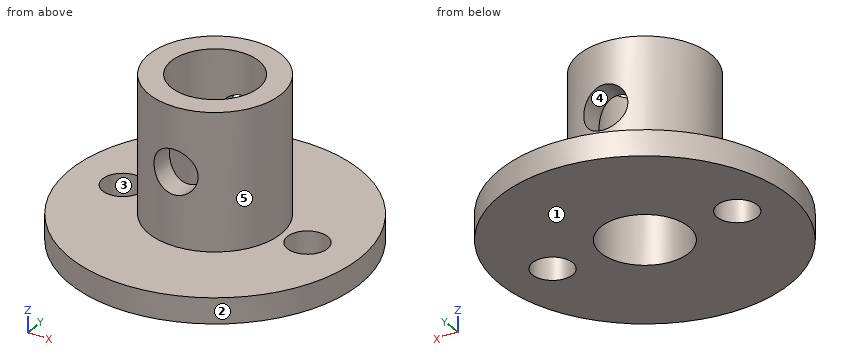
```python
from build123d import *

# Parameters (mm, degrees)
SKETCH1_W               = 10.16
SKETCH1_H               = 1.651
CUT_EXTRUDE1_DEPTH      = 20.458372876
CUT_EXTRUDE1_DEPTH_BACK = 20.458372876
SKETCH2_R               = 1.651
CUT_EXTRUDE2_DEPTH      = 19.338201985
CUT_EXTRUDE2_DEPTH_BACK = 19.338201985
SKETCH3_R               = 1.5


with BuildPart() as part:
    # Sketch1 → Revolve1 (revolve)
    with BuildSketch(Plane(origin=(0, 0, 0), x_dir=(0, 0, -1), z_dir=(1, 0, 0)), mode=Mode.PRIVATE) as revolve1_sk:
        with Locations((-6.985, 4.0894)):
            Rectangle(SKETCH1_W, SKETCH1_H)
        Polygon((-1.905, 10.795), (-1.905, 4.9149), (-1.905, 3.2639), (0, 3.2639), (0, 10.795), align=None)
    revolve(revolve1_sk.sketch.rotate(Axis((0, 0, 9.576838869), (0, 0, -1)), 90), axis=Axis((0, 0, 9.576838869), (0, 0, -1)))

    # Sketch2 → Cut-Extrude1 (cut, two sides: drawn at the far end of the back side and taken through both)
    with BuildSketch(Plane(origin=(0, 0, 0), x_dir=(1, 0, 0), z_dir=(0, 1, 0)).offset(-CUT_EXTRUDE1_DEPTH_BACK)):
        with Locations(Location((0, -7.3025, 0), (0, 0, 270))):
            Circle(SKETCH2_R)
    extrude(amount=CUT_EXTRUDE1_DEPTH + CUT_EXTRUDE1_DEPTH_BACK, mode=Mode.SUBTRACT)

    # Sketch3 → Cut-Extrude2 (cut, two sides: drawn at the far end of the back side and taken through both)
    with BuildSketch(Plane.XY.offset(1.905).offset(-CUT_EXTRUDE2_DEPTH_BACK)):
        with Locations((-6.9229, 0)):
            Circle(SKETCH3_R)
        with Locations((6.9229, 0)):
            Circle(SKETCH3_R)
    extrude(amount=CUT_EXTRUDE2_DEPTH + CUT_EXTRUDE2_DEPTH_BACK, mode=Mode.SUBTRACT)


solid = part.part
```
Source: CAD feature listing. Evaluate the final solid. Frame: model axes, mm. Face numbers are marked on the shaded views. A direction names the side the tool comes from. Round coordinates to 2 decimals unless told otherwise and drop trailing zeros. Loops run counter-clockwise (first coordinate to the right, second up) from the corner with the lowest first, then second, coordinate; pieces in that order, holes last. Notation, with made-up numbers: M 83,74 L 126,74 A11 ccw 126,83 Z; hole C -25.75,-21.5 d11. An arc over 180 degrees is marked long. Use a Markdown table: item, result. Add a question column.
1. Section query C-C on z = 9.75. Return the cut outline in (x, y), then the cut area to 3 significant figures.
2. Section query A-A on x = 0. Return the cut outline in (y, z) (1 decimal).
3. Section query B-B on y = 0. Return the cut outline in (x, z) (3 decimals).
4. Section query D-D on x = 6.25. Return the cut outline in (y, z) (3 decimals).
5. Reachability of the marked faces 4 and 5 from +Z, -Z, +X, -X, +Y, -Y: full face, straight path, thin tool, end or side. Return the list, or none.
6. Contact query for flat-ended pins moving along their axis: P1, Ø2, axis at x = 4.5, z = 1.5, coming from the -Y side; P2, Ø5.5, axis at x = 0, z = 7.3, coming from the -Y side; P3, Ø5, axis at x = 4, z = 9.5, coming from the +Y side. Output: stop coordinate, or through.
7. Mould query, pull axis X, two halves, no side actions, for the marked faces 1, 2 and 3. Classes: pulls with the +X half, pulls with the -X half, needs draft (parallel to the pull), parting line crosses it, or undercut.
8. Line query: line 1 (Z direction, x = 0, y = 3.8) (1 decimal); line 2 (X direction, y = -1, z = 1.5); line 3 (Z direction, x = 9, y = -2) (3 decimals). Output: solid intervals per line, ascending.
Reported:
| question | item | result |
|---|---|---|
| 1 | outline | C 0,0 d9.83; hole C 0,0 d6.53 |
| 1 | area | 42.4 mm² |
| 2 | outline | M -10.8,0 L -3.3,0 L -3.3,5.7 L -4.9,5.7 L -4.9,1.9 L -10.8,1.9 Z; M -4.9,9 L -3.3,9 L -3.3,12.1 L -4.9,12.1 Z; M 3.3,0 L 10.8,0 L 10.8,1.9 L 4.9,1.9 L 4.9,5.7 L 3.3,5.7 Z; M 3.3,9 L 4.9,9 L 4.9,12.1 L 3.3,12.1 Z |
| 3 | outline | M -10.795,0 L -8.423,0 L -8.423,1.905 L -10.795,1.905 Z; M -5.423,0 L -3.264,0 L -3.264,12.065 L -4.915,12.065 L -4.915,1.905 L -5.423,1.905 Z; M 3.264,0 L 5.423,0 L 5.423,1.905 L 4.915,1.905 L 4.915,12.065 L 3.264,12.065 Z; M 8.423,0 L 10.795,0 L 10.795,1.905 L 8.423,1.905 Z |
| 4 | outline | M -8.802,0 L -1.341,0 L -1.341,1.905 L -8.802,1.905 Z; M 1.341,0 L 8.802,0 L 8.802,1.905 L 1.341,1.905 Z |
| 5 | face 4 | +Y, -Y |
| 5 | face 5 | +Z |
| 6 | P1 | stops at y = -10.21 |
| 6 | P2 | stops at y = -4.91 |
| 6 | P3 | stops at y = 4.68 |
| 7 | face 1 | needs draft |
| 7 | face 2 | parting line crosses it |
| 7 | face 3 | undercut |
| 8 | line 1 | z = 0 to 5.7, 9 to 12.1 |
| 8 | line 2 | x = -10.75 to -8.04, -5.8 to -3.11, 3.11 to 5.8, 8.04 to 10.75 |
| 8 | line 3 | z = 0 to 1.905 |
